Autodesk Inventor part; units mm, degrees
ref_plane "YZ Plane" through (0, 0, 0) normal (1, 0, 0) x (0, 1, 0)
ref_plane "XZ Plane" through (0, 0, 0) normal (0, 1, 0) x (-1, 0, 0)
ref_plane "XY Plane" through (0, 0, 0) normal (0, 0, 1) x (1, 0, 0)
sketch "Skizze1" plane through (0, 0, 0) normal (0, 0, 1) x (1, 0, 0)
  line L0 (24.8274, -43.9228) -> (24.8274, -19.9228)
  line L1 (24.8274, -19.9228) -> (46.0274, -19.9228)
  line L2 (46.0274, -19.9228) -> (46.0274, -67.9228)
  line L3 (34.0274, -47.9228) -> (28.8274, -47.9228)
  line L4 (28.8274, -47.9228) -> (24.8274, -43.9228)
  line L5 (34.0274, -47.9228) -> (34.0274, -67.9228)
  line L6 (34.0274, -67.9228) -> (46.0274, -67.9228)
  point P0 (0, 0)
  dimension "d0" = 45
  dimension "d1" = 4
  dimension "d2" = 21.2
  dimension "d7" = 28
  dimension "d8" = 20
  dimension "d9" = 12
extrude "Extrusion1" add sketch "Skizze1" along normal mid plane 30
sketch "Skizze2" plane through (46.0274, -67.9228, 15) normal (1, 0, 0) x (0, 0, -1)
  line L0 (5.0357, 14) -> (5.0357, 5)
  line L1 (5.0357, 5) -> (1.5346, 0)
  line L2 (1.5346, 0) -> (28.4654, 0)
  line L3 (0, 0) -> (30, 0)
  line L4 (28.4654, 0) -> (24.9643, 5)
  line L5 (24.9643, 5) -> (24.9643, 14)
  line L6 (24.9643, 14) -> (5.0357, 14) construction
  line L7 (15, -13.5846) -> (15, 81.5074)
  arc A0 (24.9643, 14) -> (18.9643, 20) centre (18.9643, 14) ccw
  line L8 (18.9643, 20) -> (11.0357, 20)
  arc A1 (11.0357, 20) -> (5.0357, 14) centre (11.0357, 14) ccw
  point P0 (15, 67.9228)
  dimension "d19" = 5
  dimension "d21" = 6
  dimension "d22" = 20
  dimension "d23" = 35
extrude "Extrusion2" cut sketch "Skizze2" against normal through all
chamfer "Fase1" distance 3 angle 45 2 edges at (34.0274, -67.9228, -14.2327) (34.0274, -67.9228, 14.2327)
properties part number "_WT_Aufnahme_Antriebseinheit6"
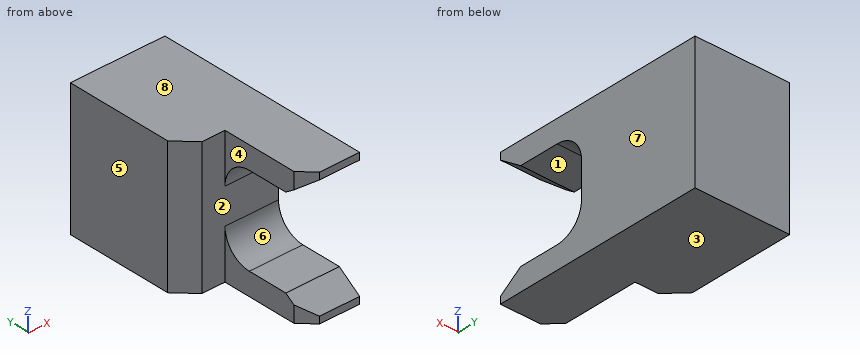
The model under review builds one solid part; all positions refer to its coordinate system, in mm. Face numbers are marked on the shaded views. A direction names the side the tool comes from. Round coordinates to 2 decimals unless told otherwise and drop trailing zeros. Loops run counter-clockwise (first coordinate to the right, second up) from the corner with the lowest first, then second, coordinate; pieces in that order, holes last. Notation, with made-up numbers: M 58.25,-37 L 106.25,-37 A30 ccw 106.25,-14 Z; hole C 56.5,-23.75 d1. An arc over 180 degrees is marked long. Put each result on its own line as item: value.
Q1. Machinability: for the marked faces 1, 2, 3, 4 and 5, which of the approach directions +Z, -Z, +X, -X, +Y, -Y give a long, thin tool a straight path to every point of the face, cutting with its end or side? Answer none if there is none.
Result set:
face 1: +X, -X, -Y
face 2: -X, -Y
face 3: -Z, +X, -X, +Y, -Y
face 4: +Z, -Z, -X, -Y
face 5: +Z, -Z, -X, +Y, -Y
Q2. Mouldability with a two-part tool opening along Z and no side actions: class the marked faces 6, 7 and 8 as released by +Z, released by -Z, zero draft, split by the parting line, or undercut.
Result set:
face 6: undercut
face 7: zero draft
face 8: released by +Z
Q3. For pin 1 (9 mm diameter, centred on y = -58, z = -11, fed in from -X); pin 2 (4 mm diameter, centred on x = 36, z = 8, fed in from -Y); pin 3 (5 mm diameter, centred on x = 41.5, z = -4.5, fed in from -Y), all flat-tipped, find the tip position at first contact; note any pin that passes through.
Result set:
pin 1: stops at x = 34.03
pin 2: stops at y = -62.97
pin 3: stops at y = -48.75
Q4. Consider section C-C, the plane z = -3.25. Give the boundary of the cut face in (x, y).
Result set:
outline: M 24.83,-43.92 L 28.83,-47.92 L 46.03,-47.92 L 46.03,-19.92 L 24.83,-19.92 Z
Q5. Consider section A-A, the plane y = -62. Give the boundary of the cut face in (x, z), then the cut area to 3 significant figures.
Result set:
outline: M 34.03,-15 L 46.03,-15 L 46.03,-9.96 L 34.03,-9.96 Z; M 34.03,9.96 L 46.03,9.96 L 46.03,15 L 34.03,15 Z
area: 121 mm²
Q6. To check wall thickness, follow L1, parallel to Y at x = 31.25, z = 3.5; L2, parallel to X at y = -51, z = -9.5; L3, parallel to Z at x = 40.5, y = -52.5. State the ranges of each line that lie inside material, in increasing order.
Result set:
L1: y = -47.92 to -19.92
L2: x = 34.03 to 46.03
L3: z = -15 to -9.79, 9.79 to 15
Q7. Consider section B-B, the plane x = 43. Give the boundary of the cut face in (y, z).
Result set:
outline: M -67.92,-15 L -19.92,-15 L -19.92,15 L -67.92,15 L -67.92,13.47 L -62.92,9.96 L -53.92,9.96 A6 cw -47.92,3.96 L -47.92,-3.96 A6 cw -53.92,-9.96 L -62.92,-9.96 L -67.92,-13.47 Z
Q8. Consider section D-D, the plane z = 12.25. Give the boundary of the cut face in (x, y).
Result set:
outline: M 24.83,-43.92 L 28.83,-47.92 L 34.03,-47.92 L 34.03,-64.92 L 35.29,-66.19 L 46.03,-66.19 L 46.03,-19.92 L 24.83,-19.92 Z
